```python
from build123d import *

# Parameters (mm, degrees)
CYLINDER011_R          = 0.6
CYLINDER011_DEPTH      = 20
BOX010_W               = 20
BOX010_H               = 5
BOX010_DEPTH           = 11
PAD001_DEPTH           = 3
SKETCH005_R            = 4
PAD002_DEPTH           = 8
SKETCH006_R            = 4
PAD003_DEPTH           = 14
BOX009_W               = 20
BOX009_H               = 5
BOX009_DEPTH           = 11
BOX009_PLACEMENT_ANGLE = 14


with BuildPart() as cylinder046:
    # Cylinder011 → Cylinder011 (new body)
    with BuildSketch(Plane(origin=(55, -9.5, -5), x_dir=(1, 0, 0), z_dir=(0, 0, 1))):
        Circle(CYLINDER011_R)
    extrude(amount=CYLINDER011_DEPTH)


with BuildPart() as cube010:
    # Box010 → Box010 (new body)
    with BuildSketch(Plane(origin=(45, -12, -0.5), x_dir=(1, 0, 0), z_dir=(0, 0, 1))):
        with Locations((10, 2.5)):
            Rectangle(BOX010_W, BOX010_H)
    extrude(amount=BOX010_DEPTH)


with BuildPart() as pad003:
    # Sketch004 → Pad001 (new body)
    with BuildSketch(Plane.XY.offset(10.5)):
        with BuildLine():
            ThreePointArc((14.120466, 10.991566), (6.522754, -2.168145), (18.163211, -11.935589))
            Line((18.163211, -11.935589), (98.163211, -11.935589))
            ThreePointArc((98.163211, -11.935589), (120.099455, 12.003546), (94.339546, 31.769884))
            Line((14.120466, 10.991566), (94.339546, 31.769884))
        make_face()
    extrude(amount=PAD001_DEPTH)

    # Sketch005 → Pad002 (new body)
    with BuildSketch(Plane(origin=(0, 0, 10.5), x_dir=(1, 0, 0), z_dir=(0, 0, -1))):
        with Locations((98.0594, -10.0638)):
            Circle(SKETCH005_R)
    extrude(amount=PAD002_DEPTH)

    # Sketch006 → Pad003 (new body)
    with BuildSketch(Plane(origin=(0, 0, 10.5), x_dir=(1, 0, 0), z_dir=(0, 0, -1))):
        with Locations((18.0594, 0)):
            Circle(SKETCH006_R)
    extrude(amount=PAD003_DEPTH)


with BuildPart() as cut010:
    # Box009 → Box009 (new body)
    with BuildSketch(Plane.XY):
        with Locations((10, 2.5)):
            Rectangle(BOX009_W, BOX009_H)
    extrude(amount=BOX009_DEPTH)


with BuildPart() as cut010_1:
    # Box009 placement: moved
    add(cut010.part.moved(Location((45, 14, -0.5))).rotate(Axis((45, 14, -0.5), (0, 0, 1)), BOX009_PLACEMENT_ANGLE))

    # Fusion005: union Cube010, Pad003
    add(cube010.part)
    add(pad003.part)

    # Cut010: cut Cylinder046
    add(cylinder046.part, mode=Mode.SUBTRACT)


solid = cut010_1.part
```
Verification items for the finished model (mm, model axes). A direction names the side the tool comes from. Give positions to 0.01 mm unless a question says otherwise; leave off trailing zeros. Loops run counter-clockwise (first coordinate to the right, second up) from the corner with the lowest first, then second, coordinate; pieces in that order, holes last. Notation, with made-up numbers: M 82,64.5 L 90,64.5 A17 ccw 90,87.5 Z; hole C -26.5,30.25 d6. An arc over 180 degrees is marked long. Return JSON: item names as keys, results as strings.
1) Section check C-C, the plane x = 32.5. Enter the section's corners in (y, z).
Findings:
{"outline": "M -11.94,10.5 L 15.75,10.5 L 15.75,13.5 L -11.94,13.5 Z"}
2) Material ranges on L1, parallel to X at y = -9.5, z = 9.5; L2, parallel to Y at x = 55, z = 7.25; L3, parallel to Z at x = 70.5, y = 12.5, recorded low to high. Write a range as [from, to].
Findings:
{"L1": "x = [45, 54.4], [55.6, 65]", "L2": "y = [-12, -10.1], [-8.9, -7], [16.49, 21.65]", "L3": "z = [10.5, 13.5]"}
3) Mould release check, pull along Y, two halves, no side actions. Record for faces 4 (the flat face through (75, 5, 10.5)), 5 (the flat face through (63.81, 21.23, 4.92)), 6 (the flat face through (45, -10, 5)): released by +Y, released by -Y, zero draft, split by the parting line, or undercut.
Findings:
{"face 4": "undercut", "face 5": "released by +Y", "face 6": "zero draft"}
4) Tool access check on faces 1 (the flat face through (55, -7, 5)), 2 (the cylindrical face through (101.754, 11.596, 6.556)), 3 (the flat face through (44.4, 16.4, 4.9)). Record the directions out of +Z, -Z, +X, -X, +Y, -Y that give a thin tool (end or side, any length) a straight path to the whole face; none if there is none.
Findings:
{"face 1": "-Z, +X, -X", "face 2": "-Z", "face 3": "-Z, -X, -Y"}
5) Section check A-A, the plane z = 11.75. Enter the section's corners in (x, y), and give its area (3 significant figures).
Findings:
{"outline": "M 14.12,10.99 A11.82 ccw 18.16,-11.94 L 98.16,-11.94 A22.02 ccw long 94.34,31.77 Z; hole C 55,-9.5 d1.2", "area": "3,730 mm2"}
6) Gauge pin test, flat ends, axial feed: P1, Ø1, axis at y = 6, z = 8.5, coming from the -X side; P2, Ø12, axis at x = 81, y = -2, coming from the -Z side; P3, Ø1.5, axis at x = 52.5, y = -9.5, coming from the -Z side; P4, Ø5, axis at x = 51.5, y = 22, coming from the +Z side. Record the tip position at first contact, or that the pin passes through.
Findings:
{"P1": "stops at x = 96.24", "P2": "stops at z = 10.5", "P3": "stops at z = -0.5", "P4": "stops at z = 13.5"}
7) Section check B-B, the plane y = 0. Enter the section's corners in (x, z).
Findings:
{"outline": "M 6.34,10.5 L 14.06,10.5 L 14.06,-3.5 L 22.06,-3.5 L 22.06,10.5 L 117.74,10.5 L 117.74,13.5 L 6.34,13.5 Z"}
8) Section check D-D, the plane y = 5. Enter the section's corners in (x, z), and give its area (3 significant figures).
Findings:
{"outline": "M 7.51,10.5 L 119.59,10.5 L 119.59,13.5 L 7.51,13.5 Z", "area": "336 mm2"}
